Verification items for the finished model (mm, model axes). Face numbers are marked on the shaded views. A direction names the side the tool comes from. Round coordinates to 2 decimals unless told otherwise and drop trailing zeros. Order: outer loops, then holes, each group sorted by start corner. A loop starts at its lowest first (then second) coordinate and runs counter-clockwise, first axis right, second up.
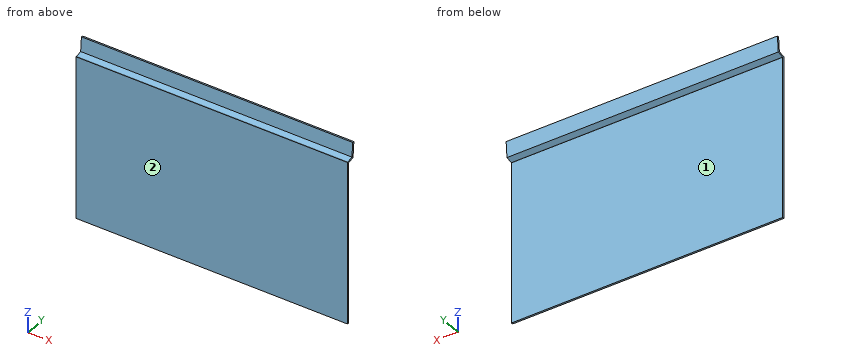
Autodesk Inventor part; units mm, degrees
ref_plane "YZ Plane" through (0, 0, 0) normal (1, 0, 0) x (0, 1, 0)
ref_plane "XZ Plane" through (0, 0, 0) normal (0, 1, 0) x (-1, 0, 0)
ref_plane "XY Plane" through (0, 0, 0) normal (0, 0, 1) x (1, 0, 0)
sketch "Sketch1" plane through (0, 0, 0) normal (1, 0, 0) x (0, 1, 0)
  line L0 (0, 0) -> (0, 597.7382)
  line L1 (0, 0) -> (3.175, 0)
  line L2 (3.175, 0) -> (3.175, 594.5632)
  line L3 (3.175, 594.5632) -> (9.906, 594.5632)
  line L4 (9.906, 594.5632) -> (15.756, 595.9828)
  line L5 (0, 597.7382) -> (9.5263, 597.7382)
  line L6 (9.5263, 597.7382) -> (12.7824, 598.5283)
  line L7 (41.2921, 902.0052) -> (15.756, 595.9828)
  line L8 (12.7824, 598.5283) -> (38.1281, 902.2692)
  line L9 (38.1281, 902.2692) -> (41.2921, 902.0052)
  line L10 (41.2921, 902.0052) -> (44.4671, 901.7403)
  line L11 (44.4671, 901.7403) -> (18.7409, 593.44)
  line L12 (18.7409, 593.44) -> (10.2857, 591.3882)
  line L13 (10.2857, 591.3882) -> (6.35, 591.3882)
  line L14 (6.35, 591.3882) -> (6.35, 574.5988)
  line L15 (6.35, 574.5988) -> (3.175, 574.5988)
  line L16 (44.4671, 901.7403) -> (47.6311, 901.4763)
  line L17 (47.6311, 901.4763) -> (21.7146, 590.8944)
  line L18 (21.7146, 590.8944) -> (10.6654, 588.2132)
  line L19 (10.6654, 588.2132) -> (9.525, 588.2132)
  line L20 (9.525, 588.2132) -> (9.525, 432.9684)
  line L21 (9.525, 432.9684) -> (6.35, 432.9684)
  line L22 (6.35, 432.9684) -> (6.35, 574.5988)
  line L23 (32.5862, 759.3601) -> (35.7502, 759.0961)
  line L24 (47.6311, 901.4763) -> (50.7951, 901.2122)
  line L25 (50.7951, 901.2122) -> (24.6882, 588.3489)
  line L26 (24.6882, 588.3489) -> (13.2454, 585.5721)
  line L27 (13.2454, 585.5721) -> (12.7, 585.5721)
  line L28 (12.7, 585.5721) -> (12.7, 289.5351)
  line L29 (23.8692, 616.7159) -> (27.0332, 616.4519)
  line L30 (12.7, 289.5351) -> (9.525, 289.5351)
  line L31 (9.525, 289.5351) -> (9.525, 432.9684)
  point P0 (14.5133, 592.4141)
  dimension "d0" = 594.5632
  dimension "d1" = 3.175
  dimension "d2" = 6.731
  dimension "d7" = 3.175
  dimension "d8" = 6.0198
  dimension "d9" = 166.36
  dimension "d10" = 3.175
  dimension "d11" = 108.41
  dimension "d12" = 3.175
  dimension "d13" = 307.086
  dimension "d18" = 3.175
  dimension "d20" = 307.1025
  dimension "d21" = 8.7006
  dimension "d22" = 3.175
  dimension "d23" = 3.175
  dimension "d24" = 3.9357
  dimension "d25" = 16.7894
  dimension "d28" = 3.175
  dimension "d29" = 3.186
  dimension "d30" = 3.175
  dimension "d32" = 3.175
  dimension "d33" = 3.175
  dimension "d34" = 142.875
  dimension "d35" = 168.7862
  dimension "d36" = 11.3698
  dimension "d37" = 1.1404
  dimension "d38" = 155.2448
  dimension "d41" = 3.175
  dimension "d42" = 3.175
  dimension "d43" = 3.175
  dimension "d44" = 142.875
  dimension "d45" = 296.037
  dimension "d46" = 28.2007
  dimension "d47" = 11.7749
  dimension "d48" = 0.5454
extrude "Extrusion4" add sketch "Sketch1" along normal blind 494.03 contours L20 L19 L18 L17 L29 L25 L26 L27 L28 L30 L31
properties part number "Third_Shingle_Over_Intake_Vent_With_Length_19.45_Inches"
1) Go/stop test with flat-tipped pins: pin 1 Ø2 at (x, y) = (222, 22) entering from -Z; pin 2 Ø0.6 at (x, y) = (159, 10) entering from +Z; pin 3 Ø1.5 at (x, z) = (201, 526.5) entering from +Y. Record where each tip stops, or that it passes through.
2) Sectioned sample at B-B on z = 508. Record the cut outline in (x, y) (3 decimals).
3) Tool access check on the marked faces 1 and 2. Record the directions out of +Z, -Z, +X, -X, +Y, -Y that give a thin tool (end or side, any length) a straight path to the whole face; none if there is none.
4) Sectioned sample at A-A on x = 131. Record the cut outline in (y, z) (3 decimals).
5) Scan lines: probe 1 along Z at (x, y) = (381, 11.5); probe 2 along Y at (x, z) = (126, 489.5) (3 decimals); probe 3 along Z at (x, y) = (68.5, 12). Record each from-to range of solid material in increasing order.
6) Sectioned sample at C-C on y = 17. Record the cut outline in (x, z).
Returned:
1. pin 1: stops at z = 587.45
1. pin 2: stops at z = 588.21
1. pin 3: stops at y = 12.7
2. outline: (0, 9.525) - (494.03, 9.525) - (494.03, 12.7) - (0, 12.7) - close
3. face 1: -Z, +X, -X, +Y
3. face 2: +Z, -Z, +X, -X, -Y
4. outline: (9.525, 289.535) - (12.7, 289.535) - (12.7, 585.572) - (13.245, 585.572) - (24.688, 588.349) - (27.033, 616.452) - (23.869, 616.716) - (21.715, 590.894) - (10.665, 588.213) - (9.525, 588.213) - close
5. probe 1: z = 289.54 to 588.42
5. probe 2: y = 9.525 to 12.7
5. probe 3: z = 289.54 to 588.54
6. outline: (0, 586.48) - (494.03, 586.48) - (494.03, 589.75) - (0, 589.75) - close
